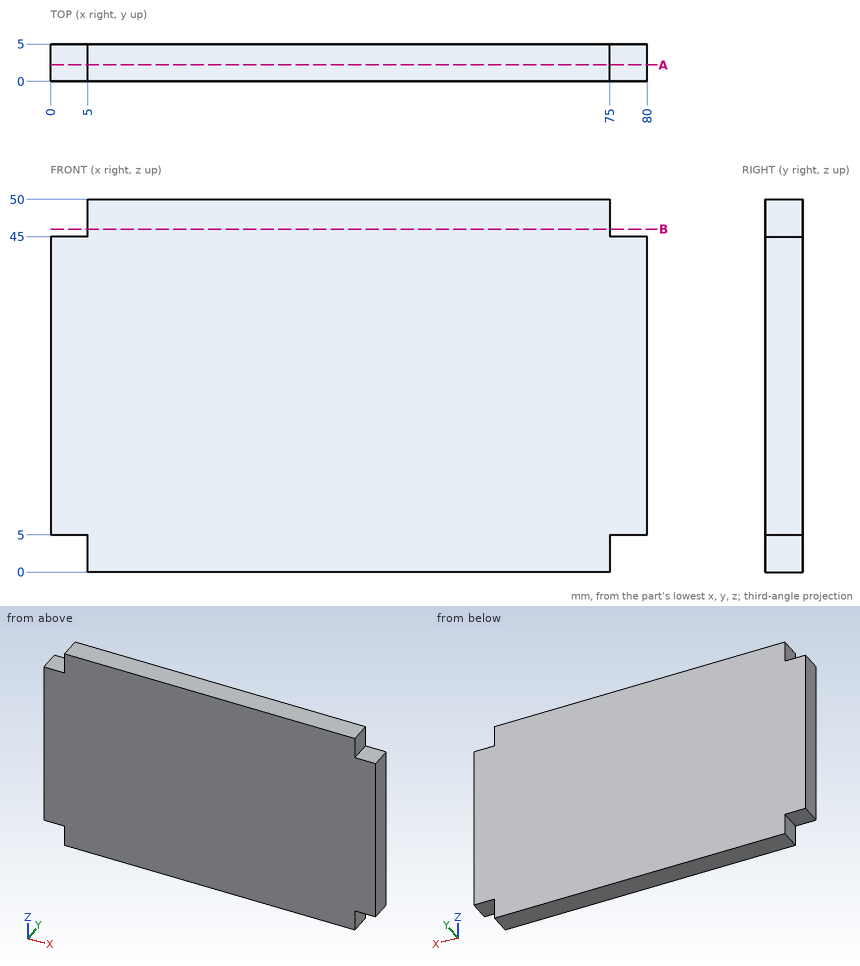
Print and shaded views of the part. All mm, measured from the part's lowest x, y and z. Coordinates: 2 decimals unless noted, no trailing zeros. Write each loop counter-clockwise with the first axis right and the second up, starting at its lowest first coordinate (ties: lowest second). Pieces come first, ordered by that corner, then holes. Notation, with made-up numbers: (76.25, 7.25) - (131.25, 7.25) arc R4 cw to (131.25, 11.25) - close; hole circle Ø2 at (50.25, 72.5). An arc over 180 degrees is marked (long way). One line per question, with ' | ' between items. Start each with the question number.
Q1. Drill centre lines: line 1 (Z direction, x = 4.5, y = 1.85); line 2 (X direction, y = 4.6, z = 4). Where is each one in solid material? Low to high. Write a range as [from, to].
Q2. Cut at B-B, the plane z = 46. List the corners of the cut face in (x, y), then the cut area to 3 significant figures.
Q3. Pin check, flat tips, straight feed: pin 1 (2.5 mm diameter, centred on x = 1.5, y = 1.5, fed in from +Z); pin 2 (1.5 mm diameter, centred on x = 2.5, y = 3, fed in from -Z). Stop position of each tip, or through.
Q4. Cut at A-A, the plane y = 2.2. List the corners of the cut face in (x, z).
Answer below:
1) line 1: [5, 45] | line 2: [5, 75]
2) outline: (5, 0) - (75, 0) - (75, 5) - (5, 5) - close | area: 350 mm^2
3) pin 1: z = 45 | pin 2: z = 5
4) outline: (0, 5) - (5, 5) - (5, 0) - (75, 0) - (75, 5) - (80, 5) - (80, 45) - (75, 45) - (75, 50) - (5, 50) - (5, 45) - (0, 45) - close
